```python
from build123d import *

# Parameters (mm, degrees)
F1_DEPTH = 20
F2_R     = 15
F3_DEPTH = 25
F4_SIZE  = 4.99999


# Not quite as in the source:
# - a fillet or chamfer is up to 0.001 mm smaller than in the source, because OpenCascade refuses the exact size


with BuildPart() as f1:
    # F0 (on Top) → F1 (new body)
    with BuildSketch(Plane.XY):
        Polygon((14.4337567297, 25), (-14.4337567297, 25), (-28.8675134595, 0), (-14.4337567297, -25), (14.4337567297, -25), (28.8675134595, 0), align=None)
    extrude(amount=F1_DEPTH)

    # F2 (on face) → F3 (cut)
    with BuildSketch(Plane.XY.offset(20)):
        Circle(F2_R)
    extrude(amount=-F3_DEPTH, mode=Mode.SUBTRACT)

    # F4 (size 5 in the source; OpenCascade refuses exactly that, so slightly less here)
    f4_edges = [f1.edges().sort_by_distance(p)[0] for p in [
        (0, 25, 20),
        (21.650635, 12.5, 20),
        (-21.650635, 12.5, 20),
        (21.650635, -12.5, 20),
        (-21.650635, -12.5, 20),
        (0, -25, 20),
        (-15, 0, 20),
        (0, 25, 0),
        (21.650635, 12.5, 0),
        (-21.650635, 12.5, 0),
        (21.650635, -12.5, 0),
        (-21.650635, -12.5, 0),
        (0, -25, 0),
        (-15, 0, 0),
    ]]
    chamfer(f4_edges, length=F4_SIZE)


solid = f1.part
```
Input: part model. Units: mm. Frame: model coordinates. Round coordinates to 2 decimals unless told otherwise and drop trailing zeros. Order: outer loops, then holes, each group sorted by start corner. A loop starts at its lowest first (then second) coordinate and runs counter-clockwise, first axis right, second up. Notation, with made-up numbers: (52.25, 24.25) - (97.25, 24.25) arc R17 cw to (97.25, 52.25) - close; hole circle Ø5 at (-2, 2.25). An arc over 180 degrees is marked (long way). One line per question, with ' | ' between items. Start each with the question number.
1) Contact query for flat-ended pins moving along their axis: P1, Ø1, axis at x = 13.5, y = -6.5, coming from the -Z side; P2, Ø1, axis at x = -19.5, z = 10, coming from the -Y side; P3, Ø8, axis at x = -21.5, z = 5, coming from the -Y side. Output: stop coordinate, or through.
2) Cut plane D-D, the plane z = 15.75. Return the cut outline in (x, y).
3) Ray query, probe 1 along Y at (x, z) = (0, 9.5); probe 2 along X at (y, z) = (-3.5, 2.5); probe 3 along Y at (x, z) = (7, 8.25). Return the intervals inside material, ascending.
4) Pull-direction query (X, two-part tool) for faces 1 (the flat face through (21.55, -12.675, 9.93)), 2 (the conical face through (14.539, 4.579, 15.243)), 3 (the flat face through (0, 22, 18)), 4 (the flat face through (-21.55, 12.675, 9.93)); classes: +X half, -X half, draft (parallel to the pull), parting line (faces both ways), or undercut.
5) Cut plane C-C, the plane y = 22.5. Return the cut outline in (x, z).
6) Cut plane B-B, the plane z = 6. Return the cut outline in (x, y).
Worked out:
1) P1: stops at z = 4.52 | P2: stops at y = -17.09 | P3: stops at y = -19.69
2) outline: (-28, 0) - (-14, -24.25) - (14, -24.25) - (28, 0) - (14, 24.25) - (-14, 24.25) - close; hole circle Ø31.5 at (0, 0)
3) probe 1: y = -25 to -15, 15 to 25 | probe 2: x = -23.96 to -17.15, 17.15 to 23.96 | probe 3: y = -25 to -13.27, 13.27 to 25
4) face 1: +X half | face 2: undercut | face 3: draft | face 4: -X half
5) outline: (-15.88, 5) - (-12.99, 2.5) - (12.99, 2.5) - (15.88, 5) - (15.88, 15) - (12.99, 17.5) - (-12.99, 17.5) - (-15.88, 15) - close
6) outline: (-28.87, 0) - (-14.43, -25) - (14.43, -25) - (28.87, 0) - (14.43, 25) - (-14.43, 25) - close; hole circle Ø30 at (0, 0)
